```python
from build123d import *

# Parameters (mm, degrees)
SKETCH1_W                                          = 12.69619
SKETCH1_H                                          = 3.556
BOSS_EXTRUDE1_DEPTH                                = 1.016
BOSS_EXTRUDE2_DEPTH                                = 2.794
SKETCH4_R                                          = 4.56565
BOSS_EXTRUDE3_DEPTH                                = 2.54
SKETCH5_R                                          = 4.56565
BOSS_EXTRUDE4_DEPTH                                = 2.54
SKETCH6_R                                          = 4.56565
BOSS_EXTRUDE5_DEPTH                                = 2.54
SKETCH7_R                                          = 4.56565
BOSS_EXTRUDE6_DEPTH                                = 2.54
HOLE1_D                                            = 12.7254
HOLE1_DEPTH                                        = 7.366
M2_5_CLEARANCE_HOLE1_D                             = 2.7051
M2_5_CLEARANCE_HOLE1_DEPTH                         = 7.366
M3_CLEARANCE_HOLE1_D                               = 3.556
M3_CLEARANCE_HOLE1_DEPTH                           = 3.556
CBORE_FOR_M2_5_HEX_HEAD_MACHINE_SCREW1_D           = 3
CBORE_FOR_M2_5_HEX_HEAD_MACHINE_SCREW1_DEPTH       = 5.334
CBORE_FOR_M2_5_HEX_HEAD_MACHINE_SCREW1_CBORE_D     = 6.35
CBORE_FOR_M2_5_HEX_HEAD_MACHINE_SCREW1_CBORE_DEPTH = 3.048


with BuildPart() as part:
    # Sketch1 → Revolve1 (revolve)
    with BuildSketch(Plane.XY):
        with Locations((6.348095, 1.778)):
            Rectangle(SKETCH1_W, SKETCH1_H)
    revolve(axis=Axis((0, 3.556, 0), (0, -1, 0)))

    # Sketch2 → Boss-Extrude1 (add)
    with BuildSketch(Plane(origin=(0, 3.556, 0), x_dir=(-1, 0, 0), z_dir=(0, 1, 0))):
        with BuildLine():
            Line((2.47008, 7.962716), (5.148593, 11.605397))
            ThreePointArc((5.148593, 11.605397), (8.977562, 8.977562), (11.605397, 5.148593))
            Line((11.605397, 5.148593), (7.962716, 2.47008))
            ThreePointArc((7.962716, 2.47008), (6.713028, 0), (7.962716, -2.47008))
            Line((7.962716, -2.47008), (11.605397, -5.148593))
            ThreePointArc((11.605397, -5.148593), (8.977562, -8.977562), (5.148593, -11.605397))
            Line((5.148593, -11.605397), (2.47008, -7.962716))
            ThreePointArc((2.47008, -7.962716), (0, -6.713028), (-2.47008, -7.962716))
            Line((-2.47008, -7.962716), (-5.148593, -11.605397))
            ThreePointArc((-5.148593, -11.605397), (-8.977562, -8.977562), (-11.605397, -5.148593))
            Line((-11.605397, -5.148593), (-7.962716, -2.47008))
            ThreePointArc((-7.962716, -2.47008), (-6.713028, 0), (-7.962716, 2.47008))
            Line((-7.962716, 2.47008), (-11.605397, 5.148593))
            ThreePointArc((-11.605397, 5.148593), (-8.977562, 8.977562), (-5.148593, 11.605397))
            Line((-5.148593, 11.605397), (-2.47008, 7.962716))
            ThreePointArc((-2.47008, 7.962716), (0, 6.713028), (2.47008, 7.962716))
        make_face()
    extrude(amount=BOSS_EXTRUDE1_DEPTH)

    # Sketch3 → Boss-Extrude2 (add)
    with BuildSketch(Plane(origin=(0, 4.572, 0), x_dir=(-1, 0, 0), z_dir=(0, 1, 0))):
        with BuildLine():
            Line((-7.962716, 2.47008), (-11.605397, 5.148593))
            Line((-11.605397, 5.148593), (-18.728402, 12.271598))
            ThreePointArc((-18.728402, 12.271598), (-18.728402, 18.728402), (-12.271598, 18.728402))
            Line((-12.271598, 18.728402), (-5.148593, 11.605397))
            Line((-5.148593, 11.605397), (-2.47008, 7.962716))
            ThreePointArc((-2.47008, 7.962716), (0, 6.713028), (2.47008, 7.962716))
            Line((2.47008, 7.962716), (5.148593, 11.605397))
            Line((5.148593, 11.605397), (12.271598, 18.728402))
            ThreePointArc((12.271598, 18.728402), (18.728402, 18.728402), (18.728402, 12.271598))
            Line((18.728402, 12.271598), (11.605397, 5.148593))
            Line((11.605397, 5.148593), (7.962716, 2.47008))
            ThreePointArc((7.962716, 2.47008), (6.713028, 0), (7.962716, -2.47008))
            Line((7.962716, -2.47008), (11.605397, -5.148593))
            Line((11.605397, -5.148593), (18.728402, -12.271598))
            ThreePointArc((18.728402, -12.271598), (18.728402, -18.728402), (12.271598, -18.728402))
            Line((12.271598, -18.728402), (5.148593, -11.605397))
            Line((5.148593, -11.605397), (2.47008, -7.962716))
            ThreePointArc((2.47008, -7.962716), (0, -6.713028), (-2.47008, -7.962716))
            Line((-2.47008, -7.962716), (-5.148593, -11.605397))
            Line((-5.148593, -11.605397), (-12.271598, -18.728402))
            ThreePointArc((-12.271598, -18.728402), (-18.728402, -18.728402), (-18.728402, -12.271598))
            Line((-18.728402, -12.271598), (-11.605397, -5.148593))
            Line((-11.605397, -5.148593), (-7.962716, -2.47008))
            ThreePointArc((-7.962716, -2.47008), (-6.713028, 0), (-7.962716, 2.47008))
        make_face()
    extrude(amount=BOSS_EXTRUDE2_DEPTH)

    # Sketch4 → Boss-Extrude3 (add)
    with BuildSketch(Plane(origin=(0, 7.366, 0), x_dir=(-1, 0, 0), z_dir=(0, 1, 0))):
        with Locations((-15.5, -15.5)):
            Circle(SKETCH4_R)
    extrude(amount=BOSS_EXTRUDE3_DEPTH)

    # Sketch5 → Boss-Extrude4 (add)
    with BuildSketch(Plane(origin=(0, 7.366, 0), x_dir=(-1, 0, 0), z_dir=(0, 1, 0))):
        with Locations((15.5, -15.5)):
            Circle(SKETCH5_R)
    extrude(amount=BOSS_EXTRUDE4_DEPTH)

    # Sketch6 → Boss-Extrude5 (add)
    with BuildSketch(Plane(origin=(0, 7.366, 0), x_dir=(-1, 0, 0), z_dir=(0, 1, 0))):
        with Locations((15.5, 15.5)):
            Circle(SKETCH6_R)
    extrude(amount=BOSS_EXTRUDE5_DEPTH)

    # Sketch7 → Boss-Extrude6 (add)
    with BuildSketch(Plane(origin=(0, 7.366, 0), x_dir=(-1, 0, 0), z_dir=(0, 1, 0))):
        with Locations((-15.5, 15.5)):
            Circle(SKETCH7_R)
    extrude(amount=BOSS_EXTRUDE6_DEPTH)

    # Hole1
    with Locations(Plane(origin=(0, 7.366, 0), x_dir=(1, 0, 0), z_dir=(0, 1, 0))):
        with Locations((0, 0)):
            Hole(HOLE1_D / 2, depth=HOLE1_DEPTH)

    # M2.5 Clearance Hole1
    with Locations(Plane(origin=(0, 7.366, 0), x_dir=(1, 0, 0), z_dir=(0, 1, 0))):
        with Locations((6.914797, -6.914797), (-6.914797, 6.914797), (6.914797, 6.914797), (-6.914797, -6.914797)):
            Hole(M2_5_CLEARANCE_HOLE1_D / 2, depth=M2_5_CLEARANCE_HOLE1_DEPTH)

    # M3 Clearance Hole1
    with Locations(Plane(origin=(0, 3.556, 0), x_dir=(1, 0, 0), z_dir=(0, 1, 0))):
        with Locations((0, -9.779), (-9.779, 0), (0, 9.779), (9.779, 0)):
            Hole(M3_CLEARANCE_HOLE1_D / 2, depth=M3_CLEARANCE_HOLE1_DEPTH)

    # CBORE for M2.5 Hex Head Machine Screw1
    with Locations(Plane(origin=(0, 4.572, 0), x_dir=(-1, 0, 0), z_dir=(0, -1, 0))):
        with Locations((-15.5, 15.5), (15.5, 15.5), (15.5, -15.5), (-15.5, -15.5)):
            CounterBoreHole(CBORE_FOR_M2_5_HEX_HEAD_MACHINE_SCREW1_D / 2, CBORE_FOR_M2_5_HEX_HEAD_MACHINE_SCREW1_CBORE_D / 2, CBORE_FOR_M2_5_HEX_HEAD_MACHINE_SCREW1_CBORE_DEPTH, depth=CBORE_FOR_M2_5_HEX_HEAD_MACHINE_SCREW1_DEPTH)


solid = part.part
```
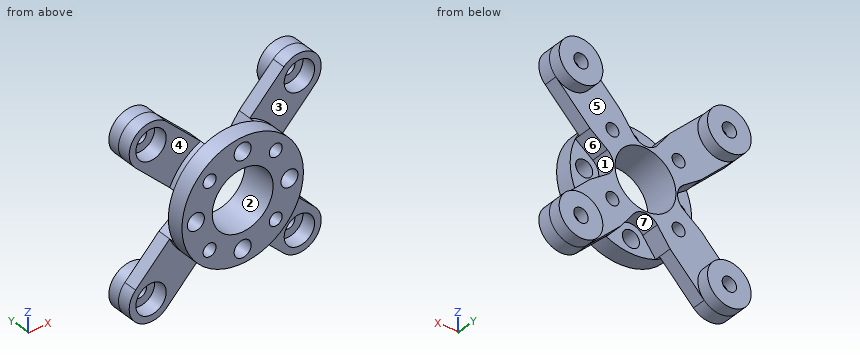
Part model, mm, in its own coordinate system. Face numbers are marked on the shaded views. A direction names the side the tool comes from. Coordinates: 2 decimals unless noted, no trailing zeros. Write each loop counter-clockwise with the first axis right and the second up, starting at its lowest first coordinate (ties: lowest second). Pieces come first, ordered by that corner, then holes.
Item 1: Which spindle directions (+Z, -Z, +X, -X, +Y, -Y) get a long thin tool onto all of the face, cutting with end or side? Do the marked faces 4, 5, 6 and 7. Say none if no direction does.
Item 2: Probe line 1 (Z direction, x = -15.5, y = 8.85); line 2 (Z direction, x = 0, y = 0.8). List the from-to ranges inside material, lowest first.
Item 3: Slice it at C-C (x = 0). Write the cut outline in (y, z).
Item 4: Pin check, flat tips, straight feed: pin 1 (1 mm diameter, centred on y = 4, z = 6, fed in from +X); pin 2 (5 mm diameter, centred on x = 15.5, z = -14.5, fed in from -Y); pin 3 (5 mm diameter, centred on x = 2, z = -11, fed in from +Y). Stop position of each tip, or through.
Item 5: Slice it at B-B (z = 0). Write the cut outline in (x, y), and give its area (3 significant figures).
Item 6: Slice it at A-A (y = 9.25). Write the cut outline in (x, z).
Item 7: Slice it at D-D (y = 1). Count the separate pieces of the cut face and the enclosed holes in it, and give its area (3 significant figures).
Item 8: Mould opens along X. For the marked faces 1, 2 and 3 say: released by +X, released by -X, zero draft, split by the parting line, or undercut.
Results found:
1. face 4: +Z, -X, -Y
1. face 5: +Y
1. face 6: +X, +Y
1. face 7: -Z, +Y
2. line 1: z = -20.07 to -17, -14 to -10.93, 10.93 to 14, 17 to 20.07
2. line 2: z = -12.7 to -11.56, -8 to -6.36, 6.36 to 8, 11.56 to 12.7
3. outline: (0, -12.7) - (3.56, -12.7) - (3.56, -11.56) - (0, -11.56) - close; (0, -8) - (3.56, -8) - (3.56, -6.71) - (7.37, -6.71) - (7.37, -6.36) - (0, -6.36) - close; (0, 6.36) - (7.37, 6.36) - (7.37, 6.71) - (3.56, 6.71) - (3.56, 8) - (0, 8) - close; (0, 11.56) - (3.56, 11.56) - (3.56, 12.7) - (0, 12.7) - close
4. pin 1: stops at x = 11.44
4. pin 2: stops at y = 4.57
4. pin 3: stops at y = 7.37
5. outline: (-12.7, 0) - (-11.56, 0) - (-11.56, 3.56) - (-12.7, 3.56) - close; (-8, 0) - (-6.36, 0) - (-6.36, 7.37) - (-6.71, 7.37) - (-6.71, 3.56) - (-8, 3.56) - close; (6.36, 0) - (8, 0) - (8, 3.56) - (6.71, 3.56) - (6.71, 7.37) - (6.36, 7.37) - close; (11.56, 0) - (12.7, 0) - (12.7, 3.56) - (11.56, 3.56) - close
5. area: 22.4 mm2
6. outline: circle Ø9.13 at (-15.5, -15.5); circle Ø9.13 at (-15.5, 15.5); circle Ø9.13 at (15.5, -15.5); circle Ø9.13 at (15.5, 15.5); hole circle Ø3 at (-15.5, -15.5); hole circle Ø3 at (-15.5, 15.5); hole circle Ø3 at (15.5, -15.5); hole circle Ø3 at (15.5, 15.5)
7. separate pieces: 1
7. enclosed holes: 9
7. area: 317 mm2
8. face 1: released by +X
8. face 2: undercut
8. face 3: zero draft
